Autodesk Inventor part; units mm, degrees
ref_plane "YZ Plane" through (0, 0, 0) normal (1, 0, 0) x (0, 1, 0)
ref_plane "XZ Plane" through (0, 0, 0) normal (0, 1, 0) x (-1, 0, 0)
ref_plane "XY Plane" through (0, 0, 0) normal (0, 0, 1) x (1, 0, 0)
sketch "Sketch1" plane through (0, 0, 0) normal (0, 0, 1) x (1, 0, 0)
  line L0 (367.7714, 50.6019) -> (367.7714, -0.1981)
  line L1 (367.7714, -0.1981) -> (367.7714, 56.9519)
  line L2 (367.7714, 56.9519) -> (367.7714, -0.1981)
  line L3 (367.7714, -0.1981) -> (43.93, -0.1981)
  line L4 (43.93, -0.1981) -> (0.2737, 43.4581)
  line L5 (0.2737, 43.4581) -> (0.2737, 56.9519)
  line L6 (0.2737, 56.9519) -> (367.7714, 56.9519)
  point P0 (0, 0)
extrude "Extrusion1" add sketch "Sketch1" along normal blind 19.05
properties part number "nd-17"
Verification items for the finished model (mm, model axes). Round coordinates to 2 decimals unless told otherwise and drop trailing zeros. Order: outer loops, then holes, each group sorted by start corner. A loop starts at its lowest first (then second) coordinate and runs counter-clockwise, first axis right, second up.
1) Material ranges on line 1 (X direction, y = 37, z = 4); line 2 (X direction, y = 27, z = 10.5); line 3 (Y direction, x = 41, z = 16.25), recorded low to high.
Geometry says:
line 1: x = 6.73 to 367.77
line 2: x = 16.73 to 367.77
line 3: y = 2.73 to 56.95
2) Cross-section at C-C, the plane y = 15. Record the cut outline in (x, z), plus the area to 3 significant figures.
Geometry says:
outline: (28.73, 0) - (367.77, 0) - (367.77, 19.05) - (28.73, 19.05) - close
area: 6,460 mm2
3) Cross-section at B-B, the plane y = 33. Record the cut outline in (x, z), plus the area to 3 significant figures.
Geometry says:
outline: (10.73, 0) - (367.77, 0) - (367.77, 19.05) - (10.73, 19.05) - close
area: 6,800 mm2
4) Cross-section at A-A, the plane z = 8.5. Record the cut outline in (x, y).
Geometry says:
outline: (0.27, 43.46) - (43.93, -0.2) - (367.77, -0.2) - (367.77, 56.95) - (0.27, 56.95) - close
5) Depth check by flat-ended pin: pin 1 (2 mm diameter, centred on y = 29.5, z = 16, fed in from -X). Enter the tip coordinate at first touch or a pass-through.
Geometry says:
pin 1: stops at x = 13.23
